Can you work these out from the model? Positions are in its coordinate system, mm. Face numbers are marked on the shaded views. A direction names the side the tool comes from. Round coordinates to 2 decimals unless told otherwise and drop trailing zeros. Order: outer loops, then holes, each group sorted by start corner. A loop starts at its lowest first (then second) coordinate and runs counter-clockwise, first axis right, second up.
Q1. If we section it at D-D (z = -51): Please give me the cut outline in (x, y), plus the area to 3 significant figures.
Q2. If we section it at B-B (x = 0): Please give me the cut outline in (y, z).
Q3. If we section it at A-A (x = -9.5): Please give me the cut outline in (y, z), plus the area to 3 significant figures.
Q4. For the marked faces 1, 2 and 3, which set-ups out of +Z, -Z, +X, -X, +Y, -Y let a thin tool reach every point of the face, with its end or its side?
Q5. If we section it at C-C (y = 32): Please give me the cut outline in (x, z), plus the area to 3 significant figures.
Q6. Will these pins go through, and if not, where does the flat tip stop? P1, Ø6.5, axis at x = -11, y = 8.5, coming from the -Z side; P2, Ø2, axis at x = 9.5, z = -52, coming from the +Y side; P3, Ø1.8, axis at x = -8.5, y = 10.5, coming from the +Z side.
Q7. If I drill on line 1 (X direction, y = 9.5, z = -67); line 2 (Z direction, x = 5.75, y = 36.5); line 3 (Y direction, x = 7.5, z = -58), over which ranges is the centre line in solid material (lowest first)?
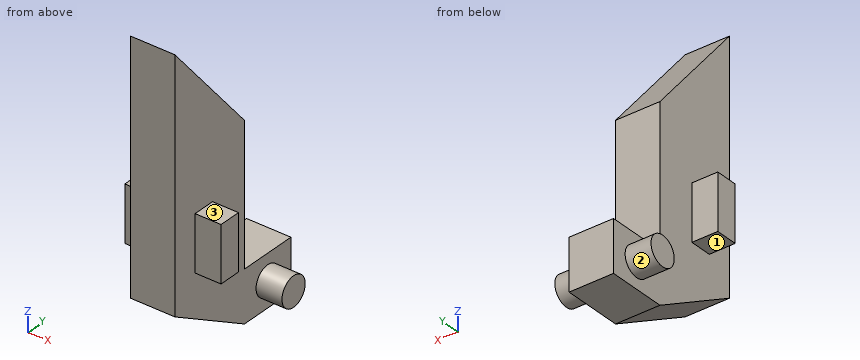
from build123d import *

# Parameters (mm, degrees)
SKETCH1_W           = 12
SKETCH1_H           = 24
BOSS_EXTRUDE1_DEPTH = 80
CUT_EXTRUDE1_DEPTH  = 52
SKETCH3_W           = 15
SKETCH3_H           = 6
BOSS_EXTRUDE2_DEPTH = 7
SKETCH4_W           = 12
SKETCH4_H           = 13.856406461
BOSS_EXTRUDE3_DEPTH = 16
SKETCH6_R           = 4
BOSS_EXTRUDE4_DEPTH = 13


with BuildPart() as part:
    # Sketch1 → Boss-Extrude1 (new body)
    with BuildSketch(Plane.XY):
        with Locations((0, 12)):
            Rectangle(SKETCH1_W, SKETCH1_H)
    extrude(amount=-BOSS_EXTRUDE1_DEPTH)

    # Sketch2 → Cut-Extrude1 (cut)
    with BuildSketch(Plane(origin=(6, 0, 0), x_dir=(0, 0, -1), z_dir=(1, 0, 0))):
        Polygon((0, 24), (0, 0), (28.602086222, 24), align=None)
        Polygon((80, 24), (66.143593539, 0), (80, 0), align=None)
    extrude(amount=-CUT_EXTRUDE1_DEPTH, mode=Mode.SUBTRACT)

    # Sketch3 → Boss-Extrude2 (add)
    with BuildSketch(Plane(origin=(6, 0, 0), x_dir=(0, 0, -1), z_dir=(1, 0, 0))):
        with Locations((51.102086222, 10)):
            Rectangle(SKETCH3_W, SKETCH3_H)
    boss_extrude2 = extrude(amount=BOSS_EXTRUDE2_DEPTH)

    # Mirror1: Boss-Extrude2 across plane
    add(boss_extrude2.mirror(Plane(origin=(0, 0, 0), x_dir=(0, 0, 1), z_dir=(1, 0, 0))))

    # Sketch4 → Boss-Extrude3 (add)
    with BuildSketch(Plane(origin=(0, 24, 0), x_dir=(1, 0, 0), z_dir=(0, 1, 0))):
        with Locations((0, 73.071796769)):
            Rectangle(SKETCH4_W, SKETCH4_H)
    extrude(amount=BOSS_EXTRUDE3_DEPTH)

    # Sketch6 → Boss-Extrude4 (add, symmetric)
    with BuildSketch(Plane(origin=(0, 0, 0), x_dir=(0, 0, -1), z_dir=(1, 0, 0))):
        with Locations(Location((73.07179677, 32, 0), (0, 0, 180))):
            Circle(SKETCH6_R)
    extrude(amount=BOSS_EXTRUDE4_DEPTH, both=True)


solid = part.part
Solution:
1. outline: (-13, 7) - (-6, 7) - (-6, 0) - (6, 0) - (6, 7) - (13, 7) - (13, 13) - (6, 13) - (6, 24) - (-6, 24) - (-6, 13) - (-13, 13) - close
1. area: 372 mm2
2. outline: (0, -66.14) - (24, -80) - (40, -80) - (40, -66.14) - (24, -66.14) - (24, -28.6) - (0, 0) - close
3. outline: (7, -58.6) - (13, -58.6) - (13, -43.6) - (7, -43.6) - close; circle Ø8 at (32, -73.07)
3. area: 140 mm2
4. face 1: -Z, -X, +Y, -Y
4. face 2: -X
4. face 3: +Z, +X, +Y, -Y
5. outline: (-13, -77.07) - (-6, -77.07) - (-6, -80) - (6, -80) - (6, -77.07) - (13, -77.07) - (13, -69.07) - (6, -69.07) - (6, -66.14) - (-6, -66.14) - (-6, -69.07) - (-13, -69.07) - close
5. area: 278 mm2
6. P1: stops at z = -58.6
6. P2: stops at y = 13
6. P3: stops at z = -43.6
7. line 1: x = -6 to 6
7. line 2: z = -80 to -66.14
7. line 3: y = 7 to 13
